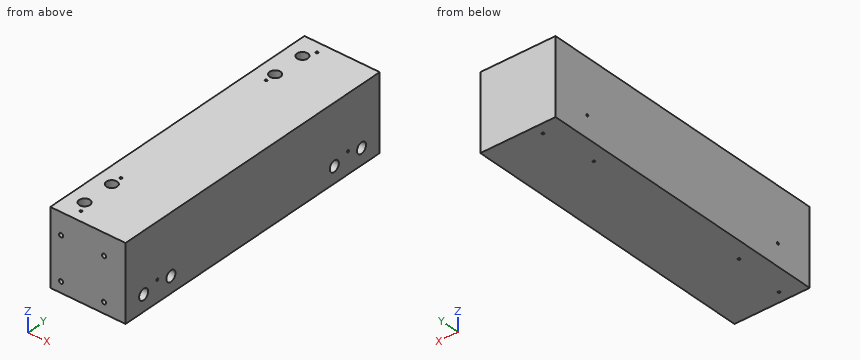
from build123d import *

# Parameters (mm, degrees)
SKETCH1_W                                = 88.9
SKETCH1_H                                = 88.9
BOSS_EXTRUDE1_DEPTH                      = 355.6
SKETCH2_R                                = 1.3890625
CUT_EXTRUDE1_DEPTH                       = 1
CUT_EXTRUDE1_DEPTH_BACK                  = 89.9
SKETCH3_R                                = 1.3890625
CUT_EXTRUDE2_DEPTH                       = 1
CUT_EXTRUDE2_DEPTH_BACK                  = 89.9
F_1_2_0_5_DIAMETER_HOLE1_D               = 12.7
F_1_2_0_5_DIAMETER_HOLE1_DEPTH           = 19.05
F_1_2_0_5_DIAMETER_HOLE1_TIP             = 3.815464931
F_1_2_0_5_DIAMETER_HOLE1_ON_FACE_2_D     = 12.7
F_1_2_0_5_DIAMETER_HOLE1_ON_FACE_2_DEPTH = 19.05
F_1_2_0_5_DIAMETER_HOLE1_ON_FACE_2_TIP   = 3.815464931
F_10_0_1935_DIAMETER_HOLE1_D             = 4.9149
F_10_0_1935_DIAMETER_HOLE1_DEPTH         = 50.8
F_10_0_1935_DIAMETER_HOLE1_TIP           = 1.476584928


with BuildPart() as part:
    # Sketch1 → Boss-Extrude1 (new body)
    with BuildSketch(Plane(origin=(0, 0, 0), x_dir=(1, 0, 0), z_dir=(0, 1, 0))):
        with Locations((44.45, -44.45)):
            Rectangle(SKETCH1_W, SKETCH1_H)
    extrude(amount=BOSS_EXTRUDE1_DEPTH)

    # Sketch2 → Cut-Extrude1 (cut, two sides)
    with BuildSketch(Plane.XY.offset(88.9)) as cut_extrude1_sk:
        with Locations((19.05, 76.2)):
            Circle(SKETCH2_R)
        with Locations((19.05, 279.4)):
            Circle(SKETCH2_R)
        with Locations((25.4, 342.9)):
            Circle(SKETCH2_R)
        with Locations((25.4, 12.7)):
            Circle(SKETCH2_R)
    extrude(amount=CUT_EXTRUDE1_DEPTH, mode=Mode.SUBTRACT)
    extrude(cut_extrude1_sk.sketch, amount=-CUT_EXTRUDE1_DEPTH_BACK, mode=Mode.SUBTRACT)

    # Sketch3 → Cut-Extrude2 (cut, two sides)
    with BuildSketch(Plane.ZY) as cut_extrude2_sk:
        with Locations((25.4, 311.15)):
            Circle(SKETCH3_R)
        with Locations((25.4, 44.45)):
            Circle(SKETCH3_R)
    extrude(amount=CUT_EXTRUDE2_DEPTH, mode=Mode.SUBTRACT)
    extrude(cut_extrude2_sk.sketch, amount=-CUT_EXTRUDE2_DEPTH_BACK, mode=Mode.SUBTRACT)

    # 1/2 (0.5) Diameter Hole1
    with Locations(Plane(origin=(19.05, 292.1, 88.9), x_dir=(1, 0, 0), z_dir=(0, 0, 1))):
        with Locations((0, 0), (0, 38.1), (0, -266.7), (0, -228.6)):
            Hole(F_1_2_0_5_DIAMETER_HOLE1_D / 2, depth=F_1_2_0_5_DIAMETER_HOLE1_DEPTH)
            with Locations((0, 0, -(F_1_2_0_5_DIAMETER_HOLE1_DEPTH + F_1_2_0_5_DIAMETER_HOLE1_TIP / 2))):  # 118° drill point
                Cone(0, F_1_2_0_5_DIAMETER_HOLE1_D / 2, F_1_2_0_5_DIAMETER_HOLE1_TIP, mode=Mode.SUBTRACT)

    # 1/2 (0.5) Diameter Hole1 on face 2
    with Locations(Plane(origin=(88.9, 63.5, 19.05), x_dir=(0, 0, 1), z_dir=(1, 0, 0))):
        with Locations((0, 0), (0, 38.1), (0, -266.7), (0, -228.6)):
            Hole(F_1_2_0_5_DIAMETER_HOLE1_ON_FACE_2_D / 2, depth=F_1_2_0_5_DIAMETER_HOLE1_ON_FACE_2_DEPTH)
            with Locations((0, 0, -(F_1_2_0_5_DIAMETER_HOLE1_ON_FACE_2_DEPTH + F_1_2_0_5_DIAMETER_HOLE1_ON_FACE_2_TIP / 2))):  # 118° drill point
                Cone(0, F_1_2_0_5_DIAMETER_HOLE1_ON_FACE_2_D / 2, F_1_2_0_5_DIAMETER_HOLE1_ON_FACE_2_TIP, mode=Mode.SUBTRACT)

    # #10 (0.1935) Diameter Hole1
    with Locations(Plane(origin=(12.7, 0, 63.5), x_dir=(0, 0, -1), z_dir=(0, -1, 0))):
        with Locations((0, 0), (0, 50.8), (50.8, 50.8), (50.8, 0)):
            Hole(F_10_0_1935_DIAMETER_HOLE1_D / 2, depth=F_10_0_1935_DIAMETER_HOLE1_DEPTH)
            with Locations((0, 0, -(F_10_0_1935_DIAMETER_HOLE1_DEPTH + F_10_0_1935_DIAMETER_HOLE1_TIP / 2))):  # 118° drill point
                Cone(0, F_10_0_1935_DIAMETER_HOLE1_D / 2, F_10_0_1935_DIAMETER_HOLE1_TIP, mode=Mode.SUBTRACT)


solid = part.part
CAD build for the part. Positions are in the model's coordinates, mm. Coordinates: 2 decimals unless noted, no trailing zeros. Answer in a Markdown table with one row per item.
1) Band-saw the part on A-A (z = 83). Give the number of separate pieces and of enclosed holes in the cut face, and give its area (3 significant figures).
Check values:
| item | result |
|---|---|
| separate pieces | 1 |
| enclosed holes | 8 |
| area | 31,100 mm2 |
2) Flat gauge pins, fed straight in: P1, Ø7.5, axis at y = 63.5, z = 19.05, coming from the +X side; P2, Ø10, axis at y = 25.4, z = 19.05, coming from the +X side; P3, Ø2.5, axis at x = 25.4, y = 12.7, coming from the +Z side. Where does each tip first touch, or does it go through?
Check values:
| item | result |
|---|---|
| P1 | x = 68.29 |
| P2 | x = 69.04 |
| P3 | through |
3) Drill centre lines: line 1 (Z direction, x = 12.7, y = 29); line 2 (Y direction, x = 74.5, z = 19.05); line 3 (Y direction, x = 19.5, z = 16.5). Where is each one in solid material? Low to high.
Check values:
| item | result |
|---|---|
| line 1 | 0 to 10.24, 15.16 to 61.04, 65.96 to 88.9 |
| line 2 | 0 to 19.05, 31.75 to 57.15, 69.85 to 285.75, 298.45 to 323.85, 336.55 to 355.6 |
| line 3 | 0 to 74.89, 77.51 to 278.09, 280.71 to 355.6 |
